from build123d import *

# Parameters (mm, degrees)
BOSS_EXTRUDE1_DEPTH                                 = 6
CUT_EXTRUDE1_DEPTH                                  = 2
SKETCH3_R                                           = 6.05
CUT_EXTRUDE2_DEPTH                                  = 3.5
SKETCH4_R                                           = 6.85
CUT_EXTRUDE3_DEPTH                                  = 0.5
CUT_EXTRUDE4_REACH                                  = 21.358
SKETCH5_R                                           = 4.5
FILLET1_R                                           = 2
SKETCH6_R                                           = 5
SKETCH6_R_2                                         = 4.5
BOSS_EXTRUDE2_DEPTH                                 = 1
CSK_FOR_M3_COUNTERSUNK_FLAT_HEAD_SCREW1_D           = 3.4
CSK_FOR_M3_COUNTERSUNK_FLAT_HEAD_SCREW1_CSINK_D     = 6.3
CSK_FOR_M3_COUNTERSUNK_FLAT_HEAD_SCREW1_CSINK_ANGLE = 90
CHAMFER1_SIZE                                       = 1


with BuildPart() as part:
    # Sketch2 → Boss-Extrude1 (new body)
    with BuildSketch(Plane(origin=(0, 0, 0), x_dir=(1, 0, 0), z_dir=(0, 1, 0))):
        with BuildLine():
            Line((-9.5, -16.5), (-9.5, 0))
            ThreePointArc((-9.5, 0), (0, 9.5), (9.5, 0))
            Line((9.5, 0), (9.5, -16.5))
            Line((9.5, -16.5), (-9.5, -16.5))
        make_face()
    extrude(amount=BOSS_EXTRUDE1_DEPTH)

    # Sketch1 → Cut-Extrude1 (cut)
    with BuildSketch(Plane(origin=(0, 0, 0), x_dir=(1, 0, 0), z_dir=(0, 1, 0))):
        with BuildLine():
            Line((-7.1, 0), (-7.1, -16.5))
            Line((-7.1, -16.5), (7.1, -16.5))
            Line((7.1, -16.5), (7.1, 0))
            ThreePointArc((7.1, 0), (0, 7.1), (-7.1, 0))
        make_face()
    extrude(amount=CUT_EXTRUDE1_DEPTH, mode=Mode.SUBTRACT)

    # Sketch3 → Cut-Extrude2 (cut)
    with BuildSketch(Plane(origin=(0, 6, 0), x_dir=(1, 0, 0), z_dir=(0, 1, 0))):
        with Locations(Location((0, 0, 0), (0, 0, 270))):
            Circle(SKETCH3_R)
    extrude(amount=-CUT_EXTRUDE2_DEPTH, mode=Mode.SUBTRACT)

    # Sketch4 → Cut-Extrude3 (cut)
    with BuildSketch(Plane(origin=(0, 6, 0), x_dir=(1, 0, 0), z_dir=(0, 1, 0))):
        with Locations(Location((0, 0, 0), (0, 0, 270))):
            Circle(SKETCH4_R)
    extrude(amount=-CUT_EXTRUDE3_DEPTH, mode=Mode.SUBTRACT)

    # Sketch5 → Cut-Extrude4 (cut, up to next)
    with BuildSketch(Plane(origin=(0, 2.5, 0), x_dir=(1, 0, 0), z_dir=(0, 1, 0)), mode=Mode.PRIVATE) as cut_extrude4_sk1:
        with Locations(Location((0, 0, 0), (0, 0, 270))):
            Circle(SKETCH5_R)
    cut_extrude4_tool1 = extrude(cut_extrude4_sk1.sketch, amount=-CUT_EXTRUDE4_REACH, mode=Mode.PRIVATE) & part.part
    add(cut_extrude4_tool1.solids().sort_by_distance((0, 2.5, 0))[0], mode=Mode.SUBTRACT)

    # Fillet1
    fillet1_edges = [part.edges().sort_by_distance(p)[0] for p in [
        (0, 2, 16.5),
    ]]
    fillet(fillet1_edges, radius=FILLET1_R)

    # Sketch6 → Boss-Extrude2 (add)
    with BuildSketch(Plane.XZ.offset(-2)):
        with Locations(Location((0, 0, 0), (0, 0, 90))):
            Circle(SKETCH6_R)
        with Locations(Location((0, 0, 0), (0, 0, 90))):
            Circle(SKETCH6_R_2, mode=Mode.SUBTRACT)
    extrude(amount=BOSS_EXTRUDE2_DEPTH)

    # CSK for M3 Countersunk Flat Head Screw1 (through all)
    with Locations(Plane(origin=(0, 6, 0), x_dir=(1, 0, 0), z_dir=(0, 1, 0))):
        with Locations((0, -11.275)):
            CounterSinkHole(CSK_FOR_M3_COUNTERSUNK_FLAT_HEAD_SCREW1_D / 2, CSK_FOR_M3_COUNTERSUNK_FLAT_HEAD_SCREW1_CSINK_D / 2, counter_sink_angle=CSK_FOR_M3_COUNTERSUNK_FLAT_HEAD_SCREW1_CSINK_ANGLE)

    # Chamfer1
    chamfer1_edges = [part.edges().sort_by_distance(p)[0] for p in [
        (9.5, 6, 8.25),
        (0, 6, -9.5),
        (9.5, 0, 8.25),
        (-9.5, 0, 8.25),
        (0, 0, -9.5),
        (-9.5, 6, 8.25),
        (9.5, 3, 16.5),
        (-9.5, 3, 16.5),
    ]]
    chamfer(chamfer1_edges, length=CHAMFER1_SIZE)


solid = part.part
Geometry check sheet. Reference: the model listing, model coordinates, mm. A direction names the side the tool comes from. Coordinates: 2 decimals unless noted, no trailing zeros. Order: outer loops, then holes, each group sorted by start corner. A loop starts at its lowest first (then second) coordinate and runs counter-clockwise, first axis right, second up. Notation, with made-up numbers: (-5.75, -15) -> (46.25, -15) arc R18 ccw to (46.25, 8) -> close; hole circle Ø11 at (0, 50.25). An arc over 180 degrees is marked (long way). Use a Markdown table: item, result. Add a question column.
1. Set-up check for faces 4 (the face through (-9, 3, 16)), 5 (the face through (1.82, 4.02, 5.77)), 6 (the face through (0.16, 0.99, -7.1)), 7 (the face through (0.1, 2.6, 15.93)): record each of +Z, -Z, +X, -X, +Y, -Y from which the full face is reachable in a straight line by a thin tool's end or side.
2. Mould release check, pull along X, two halves, no side actions. Record for faces 1 (the face through (0.369, 3.257, 12.935)), 2 (the face through (-9.5, 3, 8)), 3 (the face through (-0.209, 2.972, -9.498)): pulls with the +X half, pulls with the -X half, needs draft (parallel to the pull), parting line crosses it, or undercut.
3. Cross-section at B-B (x = 0). Give the number of separate pieces and of enclosed holes in the cut face, and give its area (3 significant figures).
4. Go/stop test with flat-tipped pins: pin 1 Ø3.5 at (x, z) = (-2.5, 0.5) entering from +Y; pin 2 Ø11 at (x, z) = (0, 0) entering from -Y. Record where each tip stops, or that it passes through.
5. Cross-section at A-A (y = 1.6). Enter the section's corners in (x, z), and give its area (3 significant figures).
6. Material ranges on L1, parallel to X at y = 1.6, z = 0; L2, parallel to Z at x = 0.75, y = 4.3; L3, parallel to Y at x = 7, z = -0.75, recorded low to high.
7. Cross-section at C-C (z = 2.5). Enter the section's corners in (x, y), and give its area (3 significant figures).
Filled sheet:
| question | item | result |
|---|---|---|
| 1 | face 4 | +Z, -X, +Y, -Y |
| 1 | face 5 | +Y |
| 1 | face 6 | -Y |
| 1 | face 7 | +Z, -Y |
| 2 | face 1 | undercut |
| 2 | face 2 | pulls with the -X half |
| 2 | face 3 | parting line crosses it |
| 3 | separate pieces | 3 |
| 3 | enclosed holes | 0 |
| 3 | area | 44.6 mm2 |
| 4 | pin 1 | through |
| 4 | pin 2 | y = 1 |
| 5 | outline | (-9.5, 0) arc R9.5 ccw to (9.5, 0) -> (9.5, 15.5) -> (8.5, 16.5) -> (7.1, 16.5) -> (7.1, 0) arc R7.1 cw to (-7.1, 0) -> (-7.1, 16.5) -> (-8.5, 16.5) -> (-9.5, 15.5) -> close; circle Ø10 at (0, 0); hole circle Ø9 at (0, 0) |
| 5 | area | 156 mm2 |
| 6 | L1 | -9.5 to -7.1, -5 to -4.5, 4.5 to 5, 7.1 to 9.5 |
| 6 | L2 | -9.47 to -6, 6 to 9.75, 12.8 to 16.5 |
| 6 | L3 | 2 to 6 |
| 7 | outline | (-9.5, 1) -> (-8.5, 0) -> (-7.1, 0) -> (-7.1, 2) -> (-4.33, 2) -> (-4.33, 1) -> (-3.74, 1) -> (-3.74, 2.5) -> (-5.51, 2.5) -> (-5.51, 5.5) -> (-6.38, 5.5) -> (-6.38, 6) -> (-8.5, 6) -> (-9.5, 5) -> close; (3.74, 1) -> (4.33, 1) -> (4.33, 2) -> (7.1, 2) -> (7.1, 0) -> (8.5, 0) -> (9.5, 1) -> (9.5, 5) -> (8.5, 6) -> (6.38, 6) -> (6.38, 5.5) -> (5.51, 5.5) -> (5.51, 2.5) -> (3.74, 2.5) -> close |
| 7 | area | 41.6 mm2 |
